For this review, take the finished solid that the model builds, in its own axes (mm). Coordinates: 2 decimals unless noted, no trailing zeros. Loops run counter-clockwise (first coordinate to the right, second up) from the corner with the lowest first, then second, coordinate; pieces in that order, holes last. Notation, with made-up numbers: M 51.5,85 L 107.5,85 A9 ccw 107.5,93 Z; hole C 22.25,54 d3. An arc over 180 degrees is marked long. Use one line per item in the form item = value.
```python
from build123d import *

# Parameters (mm, degrees)
BOSS_EXTRUDE1_DEPTH = 1.2


with BuildPart() as part:
    # Sketch1 → Boss-Extrude1 (new body)
    with BuildSketch(Plane(origin=(0, 0, 0), x_dir=(1, 0, 0), z_dir=(0, 1, 0))):
        with BuildLine():
            Line((-0.75, 7.5725), (-7.25, 7.5725))
            ThreePointArc((-7.25, 7.5725), (-7.780330086, 7.792169914), (-8, 8.3225))
            Line((-8, 8.3225), (-8, 9.3625))
            ThreePointArc((-8, 9.3625), (-7.780330086, 9.892830086), (-7.25, 10.1125))
            Line((-7.25, 10.1125), (-0.746230206, 10.1125))
            ThreePointArc((-0.746230206, 10.1125), (-0.243153345, 10.306250351), (0, 10.787396874))
            Line((0, 10.787396874), (0, 11.9025))
            ThreePointArc((0, 11.9025), (-0.219669914, 12.432830086), (-0.75, 12.6525))
            Line((-0.75, 12.6525), (-7.25, 12.6525))
            ThreePointArc((-7.25, 12.6525), (-7.780330086, 12.872169914), (-8, 13.4025))
            Line((-8, 13.4025), (-8, 14.4425))
            ThreePointArc((-8, 14.4425), (-7.780330086, 14.972830086), (-7.25, 15.1925))
            Line((-7.25, 15.1925), (-0.746230206, 15.1925))
            ThreePointArc((-0.746230206, 15.1925), (-0.243153345, 15.386250351), (0, 15.867396874))
            Line((0, 15.867396874), (0, 22.0625))
            ThreePointArc((0, 22.0625), (-0.219669914, 22.592830086), (-0.75, 22.8125))
            Line((-0.75, 22.8125), (-7.25, 22.8125))
            ThreePointArc((-7.25, 22.8125), (-7.780330086, 23.032169914), (-8, 23.5625))
            Line((-8, 23.5625), (-8, 24.6025))
            ThreePointArc((-8, 24.6025), (-7.780330086, 25.132830086), (-7.25, 25.3525))
            Line((-7.25, 25.3525), (-0.746230206, 25.3525))
            ThreePointArc((-0.746230206, 25.3525), (-0.243153345, 25.546250351), (0, 26.027396874))
            Line((0, 26.027396874), (0, 27.1425))
            ThreePointArc((0, 27.1425), (-0.219669914, 27.672830086), (-0.75, 27.8925))
            Line((-0.75, 27.8925), (-7.25, 27.8925))
            ThreePointArc((-7.25, 27.8925), (-7.780330086, 28.112169914), (-8, 28.6425))
            Line((-8, 28.6425), (-8, 29.6825))
            ThreePointArc((-8, 29.6825), (-7.780330086, 30.212830086), (-7.25, 30.4325))
            Line((-7.25, 30.4325), (-0.746230206, 30.4325))
            ThreePointArc((-0.746230206, 30.4325), (-0.243153345, 30.626250351), (0, 31.107396874))
            Line((0, 31.107396874), (0, 37.3025))
            ThreePointArc((0, 37.3025), (-0.219669914, 37.832830086), (-0.75, 38.0525))
            Line((-0.75, 38.0525), (-7.25, 38.0525))
            ThreePointArc((-7.25, 38.0525), (-7.780330086, 38.272169914), (-8, 38.8025))
            Line((-8, 38.8025), (-8, 39.8425))
            ThreePointArc((-8, 39.8425), (-7.780330086, 40.372830086), (-7.25, 40.5925))
            Line((-7.25, 40.5925), (-0.746230206, 40.5925))
            ThreePointArc((-0.746230206, 40.5925), (-0.243153345, 40.786250351), (0, 41.267396874))
            Line((0, 41.267396874), (0, 42.3825))
            ThreePointArc((0, 42.3825), (-0.219669914, 42.912830086), (-0.75, 43.1325))
            Line((-0.75, 43.1325), (-7.25, 43.1325))
            ThreePointArc((-7.25, 43.1325), (-7.780330086, 43.352169914), (-8, 43.8825))
            Line((-8, 43.8825), (-8, 44.9225))
            ThreePointArc((-8, 44.9225), (-7.780330086, 45.452830086), (-7.25, 45.6725))
            Line((-7.25, 45.6725), (-0.746230206, 45.6725))
            ThreePointArc((-0.746230206, 45.6725), (-0.243153345, 45.866250351), (0, 46.347396874))
            Line((0, 46.347396874), (0, 52.5425))
            ThreePointArc((0, 52.5425), (-0.219669914, 53.072830086), (-0.75, 53.2925))
            Line((-0.75, 53.2925), (-7.25, 53.2925))
            ThreePointArc((-7.25, 53.2925), (-7.780330086, 53.512169914), (-8, 54.0425))
            Line((-8, 54.0425), (-8, 55.0825))
            ThreePointArc((-8, 55.0825), (-7.780330086, 55.612830086), (-7.25, 55.8325))
            Line((-7.25, 55.8325), (-0.746230206, 55.8325))
            ThreePointArc((-0.746230206, 55.8325), (-0.243153345, 56.026250351), (0, 56.507396874))
            Line((0, 56.507396874), (0, 57.6225))
            ThreePointArc((0, 57.6225), (-0.219669914, 58.152830086), (-0.75, 58.3725))
            Line((-0.75, 58.3725), (-7.25, 58.3725))
            ThreePointArc((-7.25, 58.3725), (-7.780330086, 58.592169914), (-8, 59.1225))
            Line((-8, 59.1225), (-8, 60.1625))
            ThreePointArc((-8, 60.1625), (-7.780330086, 60.692830086), (-7.25, 60.9125))
            Line((-7.25, 60.9125), (-0.746230206, 60.9125))
            ThreePointArc((-0.746230206, 60.9125), (-0.243153345, 61.106250351), (0, 61.587396874))
            Line((0, 61.587396874), (0, 62.3125))
            ThreePointArc((0, 62.3125), (0.219669914, 62.842830086), (0.75, 63.0625))
            Line((0.75, 63.0625), (14.25, 63.0625))
            ThreePointArc((14.25, 63.0625), (14.780330086, 62.842830086), (15, 62.3125))
            Line((15, 62.3125), (15, 0.75))
            ThreePointArc((15, 0.75), (14.780330086, 0.219669914), (14.25, 0))
            Line((14.25, 0), (0.75, 0))
            ThreePointArc((0.75, 0), (0.219669914, 0.219669914), (0, 0.75))
            Line((0, 0.75), (0, 6.8225))
            ThreePointArc((0, 6.8225), (-0.219669914, 7.352830086), (-0.75, 7.5725))
        make_face()
    extrude(amount=BOSS_EXTRUDE1_DEPTH)


solid = part.part
```
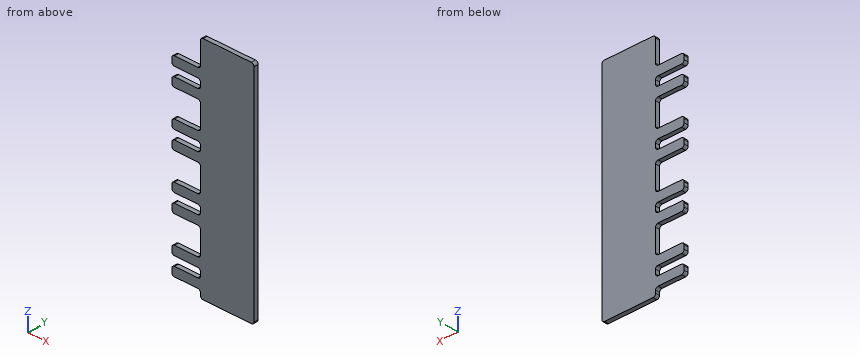
1. Consider section A-A on x = -3.25. State how many separate pieces and enclosed holes the cut face has, plus the area to 3 significant figures.
Computed values:
separate_pieces = 8
enclosed_holes = 0
area = 24.4 mm2
2. Wall thickness on line 1 along X through (y, z) = (0.55, -35); line 2 along X through (y, z) = (0.65, -40.5): over which ranges is each line inside the solid? List them lowest first. Write a range as from..to.
Computed values:
line_1 = 0..15
line_2 = -7.61..15
3. For pin 1 Ø0.6 at (x, y) = (-4, 1) entering from -Z; pin 2 Ø0.6 at (y, z) = (1, -11) entering from -X; pin 3 Ø0.6 at (x, y) = (-3.5, 0.5) entering from +Z, all flat-tipped, find the tip position at first contact; note any pin that passes through.
Computed values:
pin_1 = -60.91
pin_2 = -0.01
pin_3 = -7.57
4. Consider section B-B on z = -50.5. Write out the cut boundary in (x, y).
Computed values:
outline = M 0,0 L 15,0 L 15,1.2 L 0,1.2 Z
